from build123d import *

# Parameters (mm, degrees)
F1_DEPTH = 150


with BuildPart() as f1:
    # F0 (on Top) → F1 (new body, symmetric)
    with BuildSketch(Plane.XY):
        with BuildLine():
            Line((8.337339, -48), (6.5, -48))
            ThreePointArc((6.5, -48), (5.5, -49), (6.5, -50))
            Line((6.5, -50), (25.5, -50))
            ThreePointArc((25.5, -50), (26.914214, -49.414214), (27.5, -48))
            Line((27.5, -48), (27.5, -41.5))
            ThreePointArc((27.5, -41.5), (27.207107, -40.792893), (26.5, -40.5))
            Line((26.5, -40.5), (25.309475, -40.5))
            ThreePointArc((25.309475, -40.5), (24.955922, -40.353553), (24.809475, -40))
            Line((24.809475, -40), (24.809475, -30))
            ThreePointArc((24.809475, -30), (24.955922, -29.646447), (25.309475, -29.5))
            Line((25.309475, -29.5), (26.5, -29.5))
            ThreePointArc((26.5, -29.5), (27.207107, -29.207107), (27.5, -28.5))
            Line((27.5, -28.5), (27.5, 29))
            ThreePointArc((27.5, 29), (26.5, 30), (25.5, 29))
            Line((25.5, 29), (25.5, 24))
            ThreePointArc((25.5, 24), (25.353553, 23.646447), (25, 23.5))
            Line((25, 23.5), (20.5, 23.5))
            ThreePointArc((20.5, 23.5), (20.146447, 23.646447), (20, 24))
            Line((20, 24), (20, 47.5))
            ThreePointArc((20, 47.5), (20.146447, 47.853553), (20.5, 48))
            Line((20.5, 48), (25, 48))
            ThreePointArc((25, 48), (25.353553, 47.853553), (25.5, 47.5))
            Line((25.5, 47.5), (25.5, 42))
            ThreePointArc((25.5, 42), (26.5, 41), (27.5, 42))
            Line((27.5, 42), (27.5, 48))
            ThreePointArc((27.5, 48), (26.914214, 49.414214), (25.5, 50))
            Line((25.5, 50), (7, 50))
            ThreePointArc((7, 50), (6, 49), (7, 48))
            Line((7, 48), (17.5, 48))
            ThreePointArc((17.5, 48), (17.853553, 47.853553), (18, 47.5))
            Line((18, 47.5), (18, 40.5))
            ThreePointArc((18, 40.5), (17.853553, 40.146447), (17.5, 40))
            Line((17.5, 40), (-17.5, 40))
            ThreePointArc((-17.5, 40), (-17.853553, 40.146447), (-18, 40.5))
            Line((-18, 40.5), (-18, 47.5))
            ThreePointArc((-18, 47.5), (-17.853553, 47.853553), (-17.5, 48))
            Line((-17.5, 48), (-7, 48))
            ThreePointArc((-7, 48), (-6, 49), (-7, 50))
            Line((-7, 50), (-25.5, 50))
            ThreePointArc((-25.5, 50), (-26.914214, 49.414214), (-27.5, 48))
            Line((-27.5, 48), (-27.5, 42))
            ThreePointArc((-27.5, 42), (-26.5, 41), (-25.5, 42))
            Line((-25.5, 42), (-25.5, 47.5))
            ThreePointArc((-25.5, 47.5), (-25.353553, 47.853553), (-25, 48))
            Line((-25, 48), (-20.5, 48))
            ThreePointArc((-20.5, 48), (-20.146447, 47.853553), (-20, 47.5))
            Line((-20, 47.5), (-20, 24))
            ThreePointArc((-20, 24), (-20.146447, 23.646447), (-20.5, 23.5))
            Line((-20.5, 23.5), (-25, 23.5))
            ThreePointArc((-25, 23.5), (-25.353553, 23.646447), (-25.5, 24))
            Line((-25.5, 24), (-25.5, 29))
            ThreePointArc((-25.5, 29), (-26.5, 30), (-27.5, 29))
            Line((-27.5, 29), (-27.5, -28.5))
            ThreePointArc((-27.5, -28.5), (-27.207107, -29.207107), (-26.5, -29.5))
            Line((-26.5, -29.5), (-25.309475, -29.5))
            ThreePointArc((-25.309475, -29.5), (-24.955922, -29.646447), (-24.809475, -30))
            Line((-24.809475, -30), (-24.809475, -40))
            ThreePointArc((-24.809475, -40), (-24.955922, -40.353553), (-25.309475, -40.5))
            Line((-25.309475, -40.5), (-26.5, -40.5))
            ThreePointArc((-26.5, -40.5), (-27.207107, -40.792893), (-27.5, -41.5))
            Line((-27.5, -41.5), (-27.5, -48))
            ThreePointArc((-27.5, -48), (-26.914214, -49.414214), (-25.5, -50))
            Line((-25.5, -50), (-6.5, -50))
            ThreePointArc((-6.5, -50), (-5.5, -49), (-6.5, -48))
            Line((-6.5, -48), (-8.337339, -48))
            ThreePointArc((-8.337339, -48), (-8.690892, -47.853553), (-8.837339, -47.5))
            Line((-8.837339, -47.5), (-8.837339, -46))
            ThreePointArc((-8.837339, -46), (-8.983786, -45.646447), (-9.337339, -45.5))
            Line((-9.337339, -45.5), (-11.809584, -45.5))
            ThreePointArc((-11.809584, -45.5), (-12.0057, -45.540067), (-12.170385, -45.653846))
            ThreePointArc((-12.170385, -45.653846), (-17.986464, -47.312953), (-22.292155, -43.06555))
            ThreePointArc((-22.292155, -43.06555), (-22.305126, -43.000891), (-22.309475, -42.935087))
            Line((-22.309475, -42.935087), (-22.309475, -29.064913))
            ThreePointArc((-22.309475, -29.064913), (-22.305126, -28.999109), (-22.292155, -28.93445))
            ThreePointArc((-22.292155, -28.93445), (-18.810548, -24.962729), (-13.538514, -25.281801))
            ThreePointArc((-13.538514, -25.281801), (-12.422143, -26.044464), (-11.097021, -26.312775))
            Line((-11.097021, -26.312775), (-9.337339, -26.312775))
            ThreePointArc((-9.337339, -26.312775), (-8.983786, -26.166328), (-8.837339, -25.812775))
            Line((-8.837339, -25.812775), (-8.837339, -21.1))
            ThreePointArc((-8.837339, -21.1), (-8.36871, -19.968629), (-7.237339, -19.5))
            Line((-7.237339, -19.5), (7.237339, -19.5))
            ThreePointArc((7.237339, -19.5), (8.36871, -19.968629), (8.837339, -21.1))
            Line((8.837339, -21.1), (8.837339, -25.812775))
            ThreePointArc((8.837339, -25.812775), (8.983786, -26.166328), (9.337339, -26.312775))
            Line((9.337339, -26.312775), (11.097021, -26.312775))
            ThreePointArc((11.097021, -26.312775), (12.422143, -26.044464), (13.538514, -25.281801))
            ThreePointArc((13.538514, -25.281801), (18.810548, -24.962729), (22.292155, -28.93445))
            ThreePointArc((22.292155, -28.93445), (22.305126, -28.999109), (22.309475, -29.064913))
            Line((22.309475, -29.064913), (22.309475, -42.935087))
            ThreePointArc((22.309475, -42.935087), (22.305126, -43.000891), (22.292155, -43.06555))
            ThreePointArc((22.292155, -43.06555), (17.986464, -47.312953), (12.170385, -45.653846))
            ThreePointArc((12.170385, -45.653846), (12.0057, -45.540067), (11.809584, -45.5))
            Line((11.809584, -45.5), (9.337339, -45.5))
            ThreePointArc((9.337339, -45.5), (8.983786, -45.646447), (8.837339, -46))
            Line((8.837339, -46), (8.837339, -47.5))
            ThreePointArc((8.837339, -47.5), (8.690892, -47.853553), (8.337339, -48))
        make_face()
        with BuildLine():
            Line((25.5, 14.609856), (25.5, -14.109856))
            ThreePointArc((25.5, -14.109856), (25.293702, -14.514503), (24.845044, -14.585239))
            ThreePointArc((24.845044, -14.585239), (23.177755, -15.114626), (23.145815, -16.86365))
            ThreePointArc((23.145815, -16.86365), (21.5, -20), (19.854185, -16.86365))
            ThreePointArc((19.854185, -16.86365), (19.472086, -14.777026), (17.385462, -15.159125))
            ThreePointArc((17.385462, -15.159125), (16.504567, -18.213656), (17.643054, -21.181818))
            ThreePointArc((17.643054, -21.181818), (17.709626, -21.713201), (17.257359, -22))
            Line((17.257359, -22), (11.837339, -22))
            ThreePointArc((11.837339, -22), (11.483786, -21.853553), (11.337339, -21.5))
            Line((11.337339, -21.5), (11.337339, -21.1))
            ThreePointArc((11.337339, -21.1), (10.136477, -18.200862), (7.237339, -17))
            Line((7.237339, -17), (-7.237339, -17))
            ThreePointArc((-7.237339, -17), (-10.136477, -18.200862), (-11.337339, -21.1))
            Line((-11.337339, -21.1), (-11.337339, -21.5))
            ThreePointArc((-11.337339, -21.5), (-11.483786, -21.853553), (-11.837339, -22))
            Line((-11.837339, -22), (-17.257359, -22))
            ThreePointArc((-17.257359, -22), (-17.709626, -21.713201), (-17.643054, -21.181818))
            ThreePointArc((-17.643054, -21.181818), (-16.504567, -18.213656), (-17.385462, -15.159125))
            ThreePointArc((-17.385462, -15.159125), (-19.472086, -14.777026), (-19.854185, -16.86365))
            ThreePointArc((-19.854185, -16.86365), (-21.5, -20), (-23.145815, -16.86365))
            ThreePointArc((-23.145815, -16.86365), (-23.177755, -15.114626), (-24.845044, -14.585239))
            ThreePointArc((-24.845044, -14.585239), (-25.293702, -14.514503), (-25.5, -14.109856))
            Line((-25.5, -14.109856), (-25.5, 14.609856))
            ThreePointArc((-25.5, 14.609856), (-25.293702, 15.014503), (-24.845044, 15.085239))
            ThreePointArc((-24.845044, 15.085239), (-23.177755, 15.614626), (-23.145815, 17.36365))
            ThreePointArc((-23.145815, 17.36365), (-21.5, 20.5), (-19.854185, 17.36365))
            ThreePointArc((-19.854185, 17.36365), (-19.472086, 15.277026), (-17.385462, 15.659125))
            ThreePointArc((-17.385462, 15.659125), (-16.514462, 18.880016), (-17.863579, 21.931682))
            ThreePointArc((-17.863579, 21.931682), (-17.964645, 22.09029), (-18, 22.275009))
            Line((-18, 22.275009), (-18, 36.5))
            ThreePointArc((-18, 36.5), (-17.707107, 37.207107), (-17, 37.5))
            Line((-17, 37.5), (17, 37.5))
            ThreePointArc((17, 37.5), (17.707107, 37.207107), (18, 36.5))
            Line((18, 36.5), (18, 22.275009))
            ThreePointArc((18, 22.275009), (17.964645, 22.09029), (17.863579, 21.931682))
            ThreePointArc((17.863579, 21.931682), (16.514462, 18.880016), (17.385462, 15.659125))
            ThreePointArc((17.385462, 15.659125), (19.472086, 15.277026), (19.854185, 17.36365))
            ThreePointArc((19.854185, 17.36365), (21.5, 20.5), (23.145815, 17.36365))
            ThreePointArc((23.145815, 17.36365), (23.177755, 15.614626), (24.845044, 15.085239))
            ThreePointArc((24.845044, 15.085239), (25.293702, 15.014503), (25.5, 14.609856))
        make_face(mode=Mode.SUBTRACT)
    extrude(amount=F1_DEPTH, both=True)


solid = f1.part
Model file for the job. Use its own axes, mm. A direction names the side the tool comes from. Give positions to 0.01 mm unless a question says otherwise; leave off trailing zeros. Order: outer loops, then holes, each group sorted by start corner. A loop starts at its lowest first (then second) coordinate and runs counter-clockwise, first axis right, second up. Notation, with made-up numbers: (-16.5, 51.5) - (0.5, 51.5) arc R20 ccw to (0.5, 87.5) - close; hole circle Ø4 at (-12, -34). An arc over 180 degrees is marked (long way). Write item = value, one per line. Start each with the question number.
1. Cut at A-A, the plane y = -4.5. List the corners of the cut face in (x, z).
2. Probe line 1 along X through (y, z) = (18.5, -63); line 2 along X through (y, z) = (19, 2); line 3 along Y through (x, z) = (21, -65). List the from-to ranges inside material, lowest first.
3. Drop a flat-ended pin along its axis: P1, Ø1.5, axis at x = 1, z = -35.5, coming from the +Y side. Give the stop position or say it passes through.
4. Which spindle directions (+Z, -Z, +X, -X, +Y, -Y) get a long thin tool onto all of the face, cutting with end or side? Do faces 1 (the flat face through (27.5, 0, 2)), 2 (the flat face through (-12, 48, 2)). Say none if no direction does.
5. Two-plate mould, pull along X, no slides. Class faces 3 (the flat face through (25.5, 0, 2)), 4 (the flat face through (16, 50, 2)), 5 (the flat face through (-24.809, -35, 2)): pulls with the +X half, pulls with the -X half, needs draft (parallel to the pull), parting line crosses it, or undercut.
Taken from the geometry:
q1.outline = (-27.5, -150) - (-25.5, -150) - (-25.5, 150) - (-27.5, 150) - close; (25.5, -150) - (27.5, -150) - (27.5, 150) - (25.5, 150) - close
q2.line_1 = -27.5 to -23.5, -19.5 to -16.5, 16.5 to 19.5, 23.5 to 27.5
q2.line_2 = -27.5 to -23.44, -19.56 to -16.53, 16.53 to 19.56, 23.44 to 27.5
q2.line_3 = -50 to -45.47, -26.53 to -19.94, 20.44 to 23.5, 48 to 50
q3.P1 = 40
q4.face_1 = +Z, -Z, +X, +Y, -Y
q4.face_2 = +Z, -Z
q5.face_3 = undercut
q5.face_4 = needs draft
q5.face_5 = pulls with the -X half
